Print and shaded views of the part. All mm, measured from the part's lowest x, y and z. A direction names the side the tool comes from. Round coordinates to 2 decimals unless told otherwise and drop trailing zeros. Loops run counter-clockwise (first coordinate to the right, second up) from the corner with the lowest first, then second, coordinate; pieces in that order, holes last. Notation, with made-up numbers: (5, 64) - (14, 64) arc R6 cw to (14, 71) - close; hole circle Ø2 at (-10.5, -30). An arc over 180 degrees is marked (long way). Use one line per item in the form item = value.
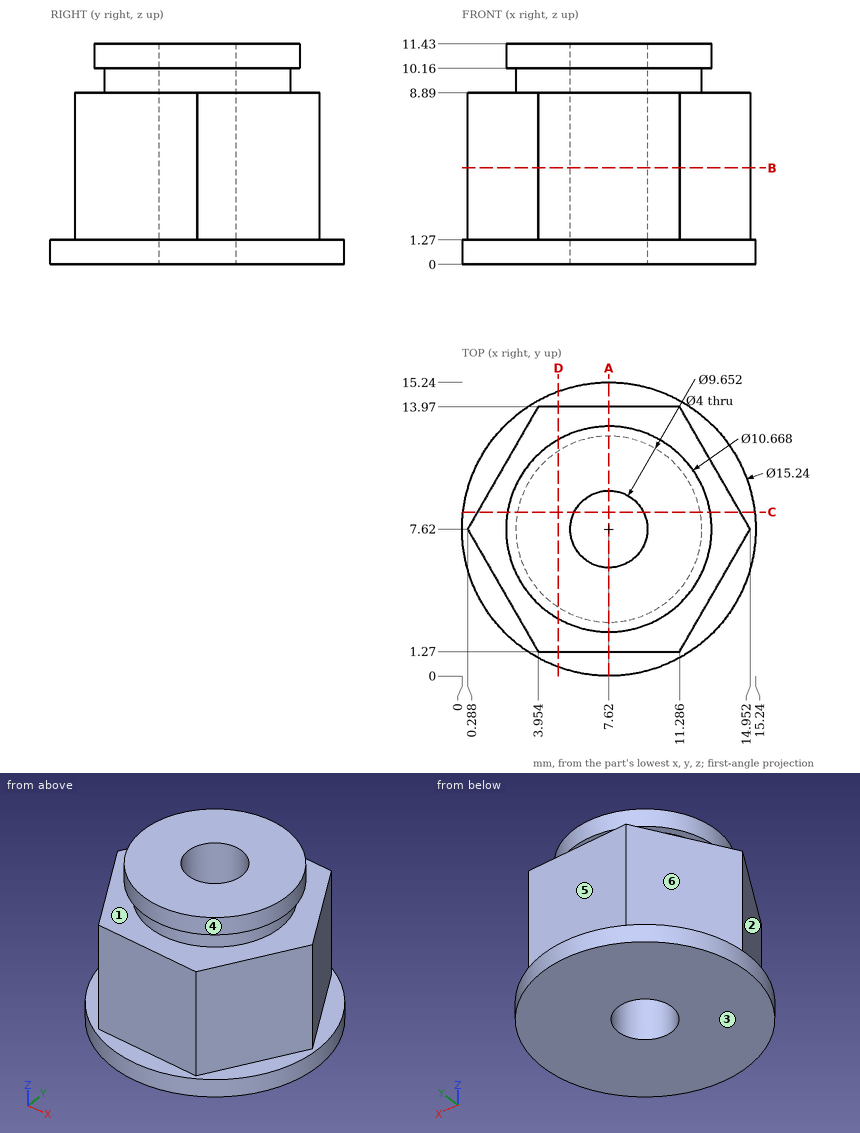
1) Slice it at D-D (x = 5). Write the cut outline in (y, z) (1 decimal), plus the area to 3 significant figures.
Report:
outline = (0.5, 0) - (14.8, 0) - (14.8, 1.3) - (14, 1.3) - (14, 8.9) - (11.7, 8.9) - (11.7, 10.2) - (12.3, 10.2) - (12.3, 11.4) - (3, 11.4) - (3, 10.2) - (3.6, 10.2) - (3.6, 8.9) - (1.3, 8.9) - (1.3, 1.3) - (0.5, 1.3) - close
area = 137 mm^2
2) Drill centre lines: probe 1 along Y at (x, z) = (7.62, 8.25); probe 2 along Z at (x, y) = (12, 11.75); probe 3 along Z at (x, y) = (6.75, 1). Where is each one in solid material? Low to high.
Report:
probe_1 = 1.27 to 5.62, 9.62 to 13.97
probe_2 = 0 to 8.89
probe_3 = 0 to 1.27
3) Two-plate mould, pull along Z, no slides. Class the marked faces 1, 2 and 3: +Z half, -Z half, draft (parallel to the pull), parting line (faces both ways), or undercut.
Report:
face_1 = undercut
face_2 = draft
face_3 = -Z half
4) Flat gauge pins, fed straight in: pin 1 (2 mm diameter, centred on x = 8.5, z = 6.5, fed in from -Y); pin 2 (3 mm diameter, centred on y = 10, z = 7.5, fed in from -X) (1 decimal); pin 3 (4 mm diameter, centred on y = 9, z = 9, fed in from +X). Where does each tip first touch, or does it go through?
Report:
pin_1 = 1.27
pin_2 = 0.8
pin_3 = 14.95
5) Slice it at A-A (x = 7.62). Write the cut outline in (y, z).
Report:
outline = (0, 0) - (5.62, 0) - (5.62, 11.43) - (2.29, 11.43) - (2.29, 10.16) - (2.79, 10.16) - (2.79, 8.89) - (1.27, 8.89) - (1.27, 1.27) - (0, 1.27) - close; (9.62, 0) - (15.24, 0) - (15.24, 1.27) - (13.97, 1.27) - (13.97, 8.89) - (12.45, 8.89) - (12.45, 10.16) - (12.95, 10.16) - (12.95, 11.43) - (9.62, 11.43) - close
6) Slice it at B-B (z = 5). Write the cut outline in (x, y), plus the area to 3 significant figures.
Report:
outline = (0.29, 7.62) - (3.95, 1.27) - (11.29, 1.27) - (14.95, 7.62) - (11.29, 13.97) - (3.95, 13.97) - close; hole circle Ø4 at (7.62, 7.62)
area = 127 mm^2
7) Slice it at C-C (y = 8.5). Write the cut outline in (x, z) (1 decimal).
Report:
outline = (0.1, 0) - (5.8, 0) - (5.8, 11.4) - (2.4, 11.4) - (2.4, 10.2) - (2.9, 10.2) - (2.9, 8.9) - (0.8, 8.9) - (0.8, 1.3) - (0.1, 1.3) - close; (9.4, 0) - (15.2, 0) - (15.2, 1.3) - (14.4, 1.3) - (14.4, 8.9) - (12.4, 8.9) - (12.4, 10.2) - (12.9, 10.2) - (12.9, 11.4) - (9.4, 11.4) - close
8) Tool access for the marked faces 4, 5 and 6: list every direction of +Z, -Z, +X, -X, +Y, -Y with a clear straight run to the whole face (end or side of a thin tool).
Report:
face_4 = +Z
face_5 = +Z, +X, -X, +Y
face_6 = +Z, -X, +Y
